Read the model definition and answer for the solid it produces. Units are mm, in the model's axes. Round coordinates to 2 decimals unless told otherwise and drop trailing zeros. Write each loop counter-clockwise with the first axis right and the second up, starting at its lowest first coordinate (ties: lowest second). Pieces come first, ordered by that corner, then holes. Notation, with made-up numbers: (-19.5, 88) -> (18.5, 88) arc R10 cw to (18.5, 101) -> close; hole circle Ø7 at (4.5, -19). An arc over 180 degrees is marked (long way). Return JSON: item names as keys, results as strings.
from build123d import *

# Parameters (mm, degrees)
SKETCH1_W             = 254
SKETCH1_H             = 55.16372
SKETCH1_R             = 13.49375
BOSS_EXTRUDE1_DEPTH   = 6.35
F_6_CLEARANCE_HOLE1_D = 3.7973
SKETCH4_W             = 165.1
SKETCH4_H             = 55.16372
CUT_EXTRUDE1_DEPTH    = 6.35
CUT_EXTRUDE2_DEPTH    = 6.35
F_6_CLEARANCE_HOLE2_D = 3.7973


with BuildPart() as part:
    # Sketch1 → Boss-Extrude1 (new body)
    with BuildSketch(Plane.XY):
        Rectangle(SKETCH1_W, SKETCH1_H)
        with Locations((-82.55, 0)):
            Circle(SKETCH1_R, mode=Mode.SUBTRACT)
        with Locations((82.55, 0)):
            Circle(SKETCH1_R, mode=Mode.SUBTRACT)
    extrude(amount=BOSS_EXTRUDE1_DEPTH)

    # #6 Clearance Hole1 (through all)
    with Locations(Plane.XY.offset(6.35)):
        with Locations((-111.76, -21.23186), (-101.6, -21.23186), (-63.5, -21.23186), (-53.34, -21.23186)):
            f_6_clearance_hole1 = Hole(F_6_CLEARANCE_HOLE1_D / 2)

    # Mirror1: #6 Clearance Hole1 across plane
    add(f_6_clearance_hole1.mirror(Plane.ZY), mode=Mode.SUBTRACT)

    # Sketch4 → Cut-Extrude1 (cut)
    with BuildSketch(Plane.XY.offset(6.35)):
        with Locations((44.45, 0)):
            Rectangle(SKETCH4_W, SKETCH4_H)
    extrude(amount=-CUT_EXTRUDE1_DEPTH, mode=Mode.SUBTRACT)

    # Sketch5 → Cut-Extrude2 (cut)
    with BuildSketch(Plane.XY.offset(6.35)):
        Polygon((-127, 3.733618756), (-101.496237284, 27.58186), (-127, 27.58186), align=None)
    extrude(amount=-CUT_EXTRUDE2_DEPTH, mode=Mode.SUBTRACT)

    # #6 Clearance Hole2 (through all)
    with Locations(Plane.XY.offset(6.35)):
        with Locations((-43.18, 23.77186), (-55.88, 23.77186), (-99.06, 23.77186), (-86.36, 23.77186)):
            Hole(F_6_CLEARANCE_HOLE2_D / 2)


solid = part.part
Item 1: A flat-ended cylindrical pin translates along its axis: pin 1 (16 mm diameter, centred on x = -82.55, y = 0, fed in from -Z). Find the tip coordinate at first contact, or state that the pin passes through.
Worked answers:
{"pin 1": "passes through"}
Item 2: Section B-B (z = 3.75) is taken. State how many separate pieces and enclosed holes the cut face has, then the cut area to 3 significant figures.
Worked answers:
{"separate pieces": "1", "enclosed holes": "9", "area": "3,940 mm2"}
Item 3: For a pull along Y with two mould halves and no side action, classify faces 1 (the flat face through (-70, 27.582, 3)), 2 (the cylindrical face through (-88.11, 23.04, 3.13)), 3 (the flat face through (-83, -27.582, 3)), 4 (the flat face through (-73, -12, 6.35)) as released by +Y, released by -Y, zero draft, split by the parting line, or undercut.
Worked answers:
{"face 1": "released by +Y", "face 2": "undercut", "face 3": "released by -Y", "face 4": "zero draft"}
Item 4: Section A-A (x = -82.55) is taken. Give the vertices of the cut face in (y, z).
Worked answers:
{"outline": "(-27.58, 0) -> (-13.49, 0) -> (-13.49, 6.35) -> (-27.58, 6.35) -> close; (13.49, 0) -> (27.58, 0) -> (27.58, 6.35) -> (13.49, 6.35) -> close"}
Item 5: Section D-D (x = -106) is taken. Give the vertices of the cut face in (y, z).
Worked answers:
{"outline": "(-27.58, 0) -> (23.37, 0) -> (23.37, 6.35) -> (-27.58, 6.35) -> close"}
Item 6: Straight lines are drawn through the part: L1, parallel to X at y = 24, z = 5; L2, parallel to Y at x = -43.18, z = 5; L3, parallel to Y at x = -63.5, z = 0.5. For each, find the intervals that lie inside material, in ascending order. Write a range as [from, to].
Worked answers:
{"L1": "x = [-105.33, -100.94], [-97.18, -88.24], [-84.48, -57.76], [-54, -45.06], [-41.3, -38.1]", "L2": "y = [-27.58, 21.87], [25.67, 27.58]", "L3": "y = [-27.58, -23.13], [-19.33, 27.58]"}
Item 7: Section C-C (y = -7.5) is taken. Give the vertices of the cut face in (x, z), then the cut area to 3 significant figures.
Worked answers:
{"outline": "(-127, 0) -> (-93.77, 0) -> (-93.77, 6.35) -> (-127, 6.35) -> close; (-71.33, 0) -> (-38.1, 0) -> (-38.1, 6.35) -> (-71.33, 6.35) -> close", "area": "422 mm2"}
